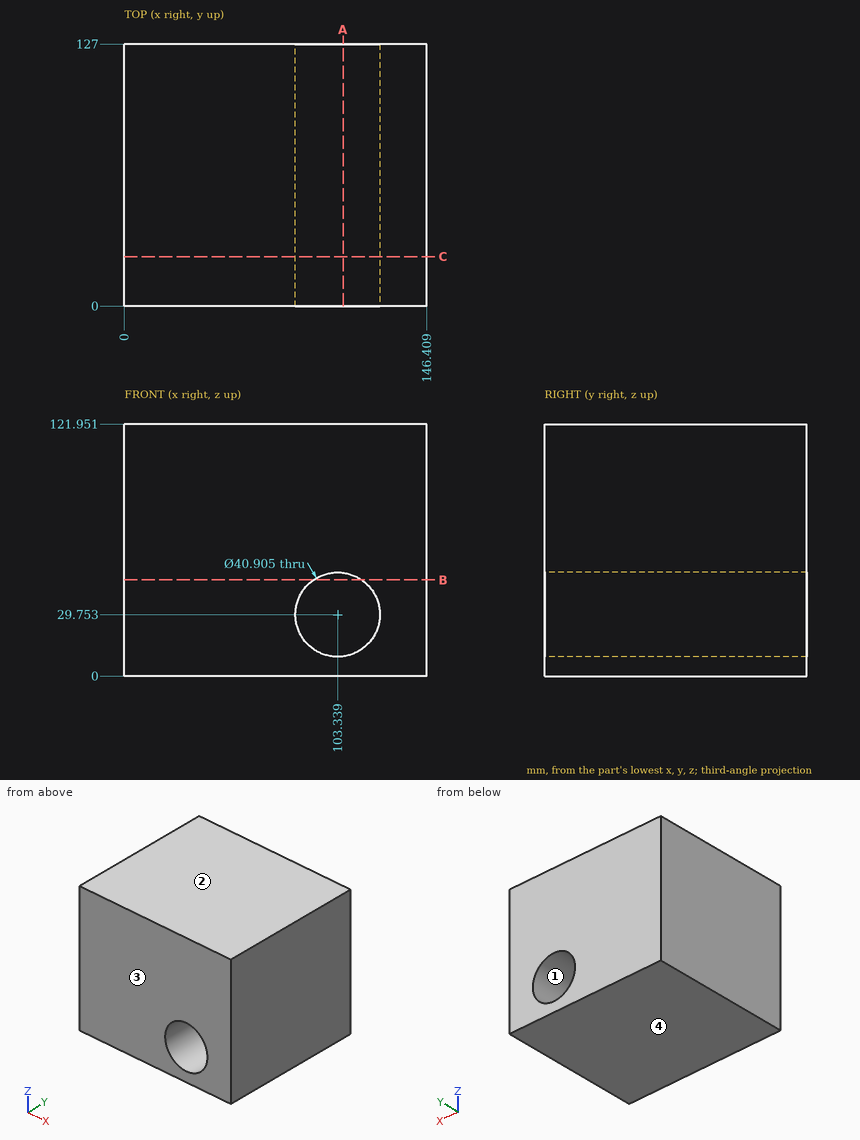
Geometry: see drawing. Coordinates: mm, zero at the bounding-box minimum. Coordinates: 2 decimals unless noted, no trailing zeros. Loops run counter-clockwise (first coordinate to the right, second up) from the corner with the lowest first, then second, coordinate; pieces in that order, holes last.
(1) Material intervals for probe 1 along Z at (x, y) = (99, 111); probe 2 along X at (y, z) = (21, 35); probe 3 along X at (y, z) = (95, 24) (1 decimal), sorted ascending.
(2) Section A-A on x = 106. Return the cut outline in (y, z) (1 decimal).
(3) Section B-B on z = 46.5. Return the cut outline in (x, y), then the cut area to 3 significant figures.
(4) Pull-direction query (Z, two-part tool) for the marked faces 1, 2, 3 and 4; classes: released by +Z, released by -Z, zero draft, split by the parting line, or undercut.
(5) Section C-C on y = 24. Return the cut outline in (x, z) (1 decimal).
Data:
1. probe 1: z = 0 to 9.77, 49.74 to 121.95
1. probe 2: x = 0 to 83.57, 123.11 to 146.41
1. probe 3: x = 0 to 83.7, 123 to 146.4
2. outline: (0, 0) - (127, 0) - (127, 9.5) - (0, 9.5) - close; (0, 50) - (127, 50) - (127, 122) - (0, 122) - close
3. outline: (0, 0) - (91.6, 0) - (91.6, 127) - (0, 127) - close; (115.08, 0) - (146.41, 0) - (146.41, 127) - (115.08, 127) - close
3. area: 15,600 mm2
4. face 1: undercut
4. face 2: released by +Z
4. face 3: zero draft
4. face 4: released by -Z
5. outline: (0, 0) - (146.4, 0) - (146.4, 122) - (0, 122) - close; hole circle Ø40.9 at (103.3, 29.8)
